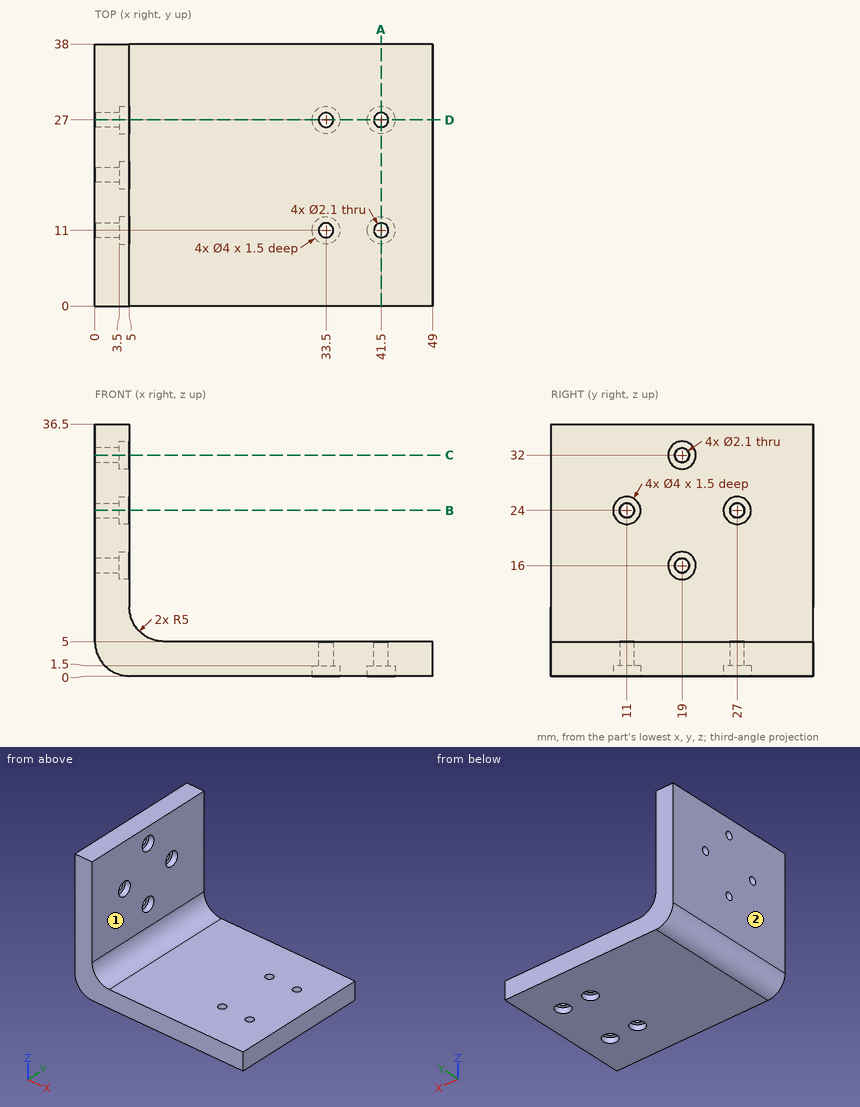
The figure shows three views and two pictorial views of one solid part (mm, origin at its lowest corner). Answer the questions. A direction names the side the tool comes from. Coordinates: 2 decimals unless noted, no trailing zeros. Loops run counter-clockwise (first coordinate to the right, second up) from the corner with the lowest first, then second, coordinate; pieces in that order, holes last. Notation, with made-up numbers: (82.25, -34.5) -> (100.25, -34.5) arc R26 cw to (100.25, -10.5) -> close; hole circle Ø2 at (53, 24). An arc over 180 degrees is marked (long way). Write item = value, one per line. Start each with the question number.
1) A cutting plane is placed at D-D (y = 27). Count the separate pieces of the cut face and the enclosed holes in it, then the cut area to 3 significant figures.
2) Straight lines are drawn through the part: line 1 (Y direction, x = 4.65, z = 24); line 2 (Z direction, x = 1.1, y = 19); line 3 (Z direction, x = 39, y = 21). For each, find the intervals that lie inside material, in ascending order. Write a range as from..to.
3) A cutting plane is placed at C-C (z = 32). Give the vertices of the cut face in (x, y).
4) A cutting plane is placed at B-B (z = 24). Give the vertices of the cut face in (x, y).
5) A cutting plane is placed at A-A (x = 41.5). Give the vertices of the cut face in (y, z), then the cut area to 3 significant figures.
6) A tool of negligible diameter and unlimited length cuts with its end or side. For the marked faces 1 and 2, from which of +Z, -Z, +X, -X, +Y, -Y can it reach the whole face along a straight path? Write none if from no direction.
7) Given pin 1 Ø1.3 at (y, z) = (19, 32) entering from -X; pin 2 Ø8 at (y, z) = (11, 24) entering from +X; pin 3 Ø2 at (y, z) = (19.5, 32) entering from +X; pin 4 Ø4 at (x, y) = (25.5, 5) entering from +Z, each flat-ended and moving along its own axis, determine where each tip first touches the part or whether it passes through.
Responses:
q1.separate_pieces = 4
q1.enclosed_holes = 0
q1.area = 362 mm²
q2.line_1 = 0..9, 13..25, 29..38
q2.line_2 = 1.87..14.95, 17.05..30.95, 33.05..36.5
q2.line_3 = 0..5
q3.outline = (0, 0) -> (5, 0) -> (5, 17) -> (3.5, 17) -> (3.5, 17.95) -> (0, 17.95) -> close; (0, 20.05) -> (3.5, 20.05) -> (3.5, 21) -> (5, 21) -> (5, 38) -> (0, 38) -> close
q4.outline = (0, 0) -> (5, 0) -> (5, 9) -> (3.5, 9) -> (3.5, 9.95) -> (0, 9.95) -> close; (0, 12.05) -> (3.5, 12.05) -> (3.5, 13) -> (5, 13) -> (5, 25) -> (3.5, 25) -> (3.5, 25.95) -> (0, 25.95) -> close; (0, 28.05) -> (3.5, 28.05) -> (3.5, 29) -> (5, 29) -> (5, 38) -> (0, 38) -> close
q5.outline = (0, 0) -> (9, 0) -> (9, 1.5) -> (9.95, 1.5) -> (9.95, 5) -> (0, 5) -> close; (12.05, 1.5) -> (13, 1.5) -> (13, 0) -> (25, 0) -> (25, 1.5) -> (25.95, 1.5) -> (25.95, 5) -> (12.05, 5) -> close; (28.05, 1.5) -> (29, 1.5) -> (29, 0) -> (38, 0) -> (38, 5) -> (28.05, 5) -> close
q5.area = 163 mm²
q6.face_1 = +Z, +X, +Y, -Y
q6.face_2 = +Z, -Z, -X, +Y, -Y
q7.pin_1 = through
q7.pin_2 = 5
q7.pin_3 = 3.5
q7.pin_4 = 5
